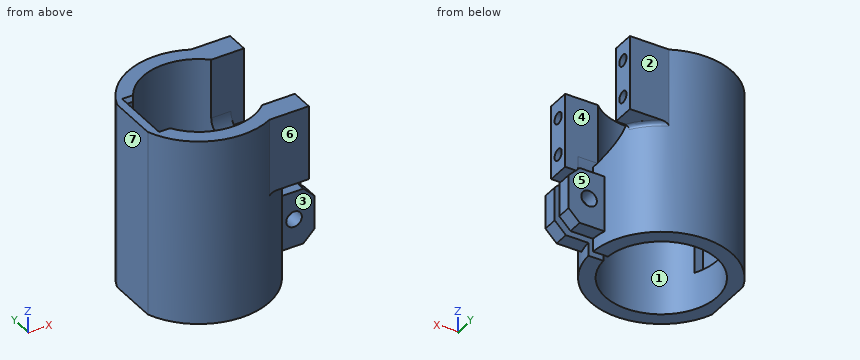
```python
from build123d import *

# Parameters (mm, degrees)
SKETCH_1_R                = 19
EXTRUDE_2_DEPTH           = 55
SKETCH_11_W               = 5
SKETCH_11_H               = 14
CUT_EXTRUDE_10_DEPTH      = 40
EXTRUDE_4_DEPTH           = 9
EXTRUDE_4_DEPTH_BACK      = 2
SKETCH_12_W               = 15
SKETCH_12_H               = 10
SKETCH_13_R               = 2.1
CUT_EXTRUDE_11_DEPTH      = 67.219332525
SKETCH_19_R               = 19
CUT_EXTRUDE_17_DEPTH      = 5
CUT_EXTRUDE_19_DEPTH      = 61.373835392
CUT_EXTRUDE_20_DEPTH      = 47.230401253
CUT_EXTRUDE_20_DEPTH_BACK = 47.230401253
SKETCH_14_W               = 20
SKETCH_14_H               = 2
CUT_EXTRUDE_21_DEPTH      = 10
SKETCH_24_W               = 20
SKETCH_24_H               = 6
EXTRUDE_5_DEPTH           = 20
SKETCH_3_R                = 15
CUT_EXTRUDE_1_DEPTH       = 61.373835507
CHAMFER_2_SIZE            = 3
CHAMFER_3_SIZE            = 1
FILLET_2_R                = 1
SKETCH_25_R               = 1.55
CUT_EXTRUDE_22_DEPTH      = 8
PATTERN_LINEAR_1_COUNT    = 2
PATTERN_LINEAR_1_PITCH    = 10
MIRROR_2_COPY_1_SKETCH_R  = 1.55
MIRROR_2_COPY_1_DEPTH     = 8
MIRROR_2_COPY_2_SKETCH_R  = 1.55
MIRROR_2_COPY_2_DEPTH     = 8
FILLET_2_OF_MIRROR_2_R    = 1


with BuildPart() as part:
    # 草圖1 → 填料-伸長2 (new body)
    with BuildSketch(Plane.XY):
        Circle(SKETCH_1_R)
    extrude(amount=EXTRUDE_2_DEPTH)

    # 草圖11 → 除料-伸長10 (cut)
    with BuildSketch(Plane.XY.offset(55)):
        with Locations((-13.1, 0)):
            Rectangle(SKETCH_11_W, SKETCH_11_H)
    extrude(amount=-CUT_EXTRUDE_10_DEPTH, mode=Mode.SUBTRACT)

    # 草圖12 → 填料-伸長4 (add, two sides: drawn at the far end of the back side and taken through both)
    with BuildSketch(Plane(origin=(19, 0, 0), x_dir=(0, 0, -1), z_dir=(1, 0, 0)).offset(-EXTRUDE_4_DEPTH_BACK)):
        with Locations((-16, 0)):
            Rectangle(SKETCH_12_W, SKETCH_12_H)
    extrude(amount=EXTRUDE_4_DEPTH + EXTRUDE_4_DEPTH_BACK)

    # 草圖13 → 除料-伸長11 (cut, through all)
    with BuildSketch(Plane.XZ.offset(5)):
        with Locations(Location((22.5, 16, 0), (0, 0, 270))):
            Circle(SKETCH_13_R)
    extrude(amount=-CUT_EXTRUDE_11_DEPTH, mode=Mode.SUBTRACT)

    # 草圖19 → 除料-伸長17 (cut)
    with BuildSketch(Plane(origin=(0, 0, 0), x_dir=(-1, 0, 0), z_dir=(0, 0, -1))):
        Circle(SKETCH_19_R)
    extrude(amount=-CUT_EXTRUDE_17_DEPTH, mode=Mode.SUBTRACT)

    # 草圖22 → 除料-伸長19 (cut, through all)
    with BuildSketch(Plane(origin=(0, 0, 5), x_dir=(-1, 0, 0), z_dir=(0, 0, -1))):
        with BuildLine():
            Line((17.8, 6.64529909), (17.8, -6.64529909))
            ThreePointArc((17.8, -6.64529909), (19, 0), (17.8, 6.64529909))
        make_face()
    extrude(amount=-CUT_EXTRUDE_19_DEPTH, mode=Mode.SUBTRACT)

    # 草圖14 → 除料-伸長20 (cut, two sides: drawn at the far end of the back side and taken through both)
    with BuildSketch(Plane.XY.offset(23.5).offset(-CUT_EXTRUDE_20_DEPTH_BACK)):
        with Locations((23.16515139, 0)):
            Rectangle(SKETCH_14_W, SKETCH_14_H)
    extrude(amount=CUT_EXTRUDE_20_DEPTH + CUT_EXTRUDE_20_DEPTH_BACK, mode=Mode.SUBTRACT)

    # 草圖23 → 除料-伸長21 (cut)
    with BuildSketch(Plane(origin=(19, 0, 0), x_dir=(0, 0, -1), z_dir=(1, 0, 0))):
        with BuildLine():
            Line((-39, 11), (-55, 11))
            Line((-55, 11), (-55, -11))
            Line((-55, -11), (-39, -11))
            ThreePointArc((-39, -11), (-28, 0), (-39, 11))
        make_face()
    extrude(amount=-CUT_EXTRUDE_21_DEPTH, mode=Mode.SUBTRACT)

    # 草圖24 → 填料-伸長5 (add)
    with BuildSketch(Plane(origin=(19, 0, 0), x_dir=(0, 0, -1), z_dir=(1, 0, 0))):
        with Locations((-45, 14)):
            Rectangle(SKETCH_24_W, SKETCH_24_H)
    extrude_5 = extrude(amount=-EXTRUDE_5_DEPTH)

    # 草圖3 → 除料-伸長1 (cut, through all)
    with BuildSketch(Plane.XY.offset(55)):
        Circle(SKETCH_3_R)
    cut_extrude_1 = extrude(amount=-CUT_EXTRUDE_1_DEPTH, mode=Mode.SUBTRACT)

    # 導角2
    chamfer_2_edges = [part.edges().sort_by_distance(p)[0] for p in [
        (28, 3, 23.5),
        (28, -3, 8.5),
        (28, -3, 23.5),
        (28, 3, 8.5),
    ]]
    chamfer(chamfer_2_edges, length=CHAMFER_2_SIZE)

    # 導角3
    chamfer_3_edges = [part.edges().sort_by_distance(p)[0] for p in [
        (-14.433249581, 7, 55),
        (-14.433249581, -7, 55),
    ]]
    chamfer(chamfer_3_edges, length=CHAMFER_3_SIZE)

    # 圓角2
    fillet_2_edges = [part.edges().sort_by_distance(p)[0] for p in [
        (12.35826472, 14.431676725, 35),
    ]]
    fillet(fillet_2_edges, radius=FILLET_2_R)

    # 草圖25 → 除料-伸長22 (cut)
    with BuildSketch(Plane(origin=(19, 0, 0), x_dir=(0, 0, -1), z_dir=(1, 0, 0))):
        with Locations((-50, 14)):
            Circle(SKETCH_25_R)
    cut_extrude_22 = extrude(amount=-CUT_EXTRUDE_22_DEPTH, mode=Mode.SUBTRACT)

    # 直線複製排列1: 除料-伸長22 ×2
    with Locations(*[(0, 0, -i * PATTERN_LINEAR_1_PITCH) for i in range(1, PATTERN_LINEAR_1_COUNT)]):
        add(cut_extrude_22, mode=Mode.SUBTRACT)

    # 鏡射2: 填料-伸長5, 除料-伸長1 across plane
    add(extrude_5.mirror(Plane.ZX))
    add(cut_extrude_1.mirror(Plane.ZX), mode=Mode.SUBTRACT)

    # 鏡射2 copy 1 sketch → 鏡射2 copy 1 (cut)
    with BuildSketch(Plane(origin=(19, 0, -10), x_dir=(0, 0, -1), z_dir=(1, 0, 0))):
        with Locations((-50, -14)):
            Circle(MIRROR_2_COPY_1_SKETCH_R)
    extrude(amount=-MIRROR_2_COPY_1_DEPTH, mode=Mode.SUBTRACT)

    # 鏡射2 copy 2 sketch → 鏡射2 copy 2 (cut)
    with BuildSketch(Plane(origin=(19, 0, 0), x_dir=(0, 0, -1), z_dir=(1, 0, 0))):
        with Locations((-50, -14)):
            Circle(MIRROR_2_COPY_2_SKETCH_R)
    extrude(amount=-MIRROR_2_COPY_2_DEPTH, mode=Mode.SUBTRACT)

    # 圓角2 of 鏡射2
    fillet_2_of_mirror_2_edges = [part.edges().sort_by_distance(p)[0] for p in [
        (12.35826472, -14.431676725, 35),
    ]]
    fillet(fillet_2_of_mirror_2_edges, radius=FILLET_2_OF_MIRROR_2_R)


solid = part.part
```
Source: CAD feature listing. Evaluate the final solid. Frame: model axes, mm. Face numbers are marked on the shaded views. A direction names the side the tool comes from. Give positions to 0.01 mm unless a question says otherwise; leave off trailing zeros. Loops run counter-clockwise (first coordinate to the right, second up) from the corner with the lowest first, then second, coordinate; pieces in that order, holes last. Notation, with made-up numbers: (-22, -33) -> (11, -33) arc R16 cw to (11, -25) -> close; hole circle Ø6 at (-25, -32.75). An arc over 180 degrees is marked (long way). Use a Markdown table: item, result. Add a question column.
(1) Section query D-D (z = 17). Output: boundary loops of the cut face in (x, y).
(2) First-contact query: pin 1 Ø2.5 at (x, z) = (-15, 42.5) entering from -Y; pin 2 Ø3 at (y, z) = (-14, 40) entering from +X; pin 3 Ø8 at (x, z) = (20, 49) entering from -Y; pin 4 Ø4 at (x, z) = (22.5, 16) entering from +Y. Flat tips, straight axial feed; report the tip coordinate or a pass-through.
(3) Section query B-B (x = 0). Output: boundary loops of the cut face in (y, z).
(4) Pull-direction query (Y, two-part tool) for the marked faces 1, 2, 3 and 4; classes: +Y half, -Y half, draft (parallel to the pull), parting line (faces both ways), or undercut.
(5) Ray query, line 1 (Y direction, x = 14, z = 40); line 2 (X direction, y = 2, z = 16); line 3 (Y direction, x = 16, z = 46). Return the intervals inside material, ascending.
(6) Access query for the marked faces 5, 6 and 7. Directions: +Z, -Z, +X, -X, +Y, -Y. A direction counts if a zero-diameter tool reaches every point of the face in a straight line with its end or side. Return the directions, or none.
(7) Section query C-C (z = 50). Output: boundary loops of the cut face in (x, y), then the cut area to 3 significant figures.
(8) Section query A-A (y = 2.5). Output: boundary loops of the cut face in (x, z).
Checked values:
| question | item | result |
|---|---|---|
| 1 | outline | (-17.8, -6.65) arc R19 ccw to (18.33, -5) -> (20.65, -5) -> (20.65, -1) -> (14.97, -1) arc R15 cw to (-13.27, -7) -> (-15.6, -7) -> (-15.6, 7) -> (-13.27, 7) arc R15 cw to (14.97, 1) -> (20.65, 1) -> (20.65, 5) -> (18.33, 5) arc R19 ccw to (-17.8, 6.65) -> close; (24.35, -5) -> (28, -5) -> (28, -1) -> (24.35, -1) -> close; (24.35, 1) -> (28, 1) -> (28, 5) -> (24.35, 5) -> close |
| 2 | pin 1 | y = -13.11 |
| 2 | pin 2 | x = 11 |
| 2 | pin 3 | y = -17 |
| 2 | pin 4 | through |
| 3 | outline | (-19, 5) -> (-15, 5) -> (-15, 55) -> (-19, 55) -> close; (15, 5) -> (19, 5) -> (19, 55) -> (15, 55) -> close |
| 4 | face 1 | undercut |
| 4 | face 2 | +Y half |
| 4 | face 3 | -Y half |
| 4 | face 4 | undercut |
| 5 | line 1 | -17 to -15.55, -12.45 to -11, 11 to 12.45, 15.55 to 17 |
| 5 | line 2 | -17.8 to -15.6, 14.87 to 20.4, 24.6 to 28 |
| 5 | line 3 | -17 to -11, 11 to 17 |
| 6 | face 5 | +Z, -Z, +X, +Y |
| 6 | face 6 | +Z, -Z, +X, -Y |
| 6 | face 7 | +Z, -Z, -X, +Y, -Y |
| 7 | outline | (-17.8, -6.65) arc R19 ccw to (8.49, -17) -> (19, -17) -> (19, -15.55) -> (11, -15.55) -> (11, -12.45) -> (19, -12.45) -> (19, -11) -> (10.2, -11) arc R15 cw to (-13.27, -7) -> (-15.6, -7) -> (-15.6, 7) -> (-13.27, 7) arc R15 cw to (10.2, 11) -> (19, 11) -> (19, 12.45) -> (11, 12.45) -> (11, 15.55) -> (19, 15.55) -> (19, 17) -> (8.49, 17) arc R19 ccw to (-17.8, 6.65) -> close |
| 7 | area | 332 mm^2 |
| 8 | outline | (-17.8, 5) -> (-14.79, 5) -> (-14.79, 15) -> (-15.6, 15) -> (-15.6, 55) -> (-17.8, 55) -> close; (14.79, 5) -> (18.83, 5) -> (18.83, 8.5) -> (25, 8.5) -> (28, 11.5) -> (28, 20.5) -> (25, 23.5) -> (18.83, 23.5) -> (18.83, 28.29) -> (14.79, 28.29) -> close; hole circle Ø4.2 at (22.5, 16) |
